Here's how the part is built. I have some questions about the finished solid (model axes, mm). Round coordinates to 2 decimals unless told otherwise and drop trailing zeros. Loops run counter-clockwise (first coordinate to the right, second up) from the corner with the lowest first, then second, coordinate; pieces in that order, holes last. Notation, with made-up numbers: M -5,-28 L 25,-28 A13 ccw 25,-3 Z; hole C 85.25,-36 d4. An arc over 180 degrees is marked long. Answer as a JSON object with one key per item and string values.
from build123d import *

# Parameters (mm, degrees)
F0_R     = 4.7625
F1_DEPTH = 58.166
F2_R     = 2.0828
F3_DEPTH = 11.43
F5_R     = 1.1811
F6_DEPTH = 10.16
F7_SIZE  = 0.762


with BuildPart() as f1:
    # F0 (on Front) → F1 (new body)
    with BuildSketch(Plane.XZ):
        Circle(F0_R)
    extrude(amount=F1_DEPTH)

    # F2 (on face) → F3 (cut)
    with BuildSketch(Plane.XZ.offset(58.166)):
        Circle(F2_R)
    extrude(amount=-F3_DEPTH, mode=Mode.SUBTRACT)

    # F5 (on offset) → F6 (cut)
    with BuildSketch(Plane.YZ.offset(4.7879)):
        with Locations((-3.175, 0)):
            Circle(F5_R)
    extrude(amount=-F6_DEPTH, mode=Mode.SUBTRACT)

    # F7
    f7_edges = [f1.edges().sort_by_distance(p)[0] for p in [
        (-4.7625, 0, 0),
    ]]
    chamfer(f7_edges, length=F7_SIZE)


solid = f1.part
Item 1: For P1, Ø2, axis at x = 3.5, y = -16.5, coming from the +Z side; P2, Ø3.5, axis at x = 0, z = 0, coming from the -Y side; P3, Ø1.5, axis at x = -1, y = -21.5, coming from the +Z side, each with a flat end and sliding along its axis, tell me the tip position at first contact or that it passes through.
Solution:
{"P1": "stops at z = 4.05", "P2": "stops at y = -46.74", "P3": "stops at z = 4.76"}
Item 2: I want a section at A-A on z = 0. List the corners of the cut face in (x, y) for me, plus the area to 3 significant figures.
Solution:
{"outline": "M -4.76,-58.17 L -2.08,-58.17 L -2.08,-46.74 L 2.08,-46.74 L 2.08,-58.17 L 4.76,-58.17 L 4.76,-4.36 L -4.76,-4.36 Z; M -4.76,-1.99 L 4.76,-1.99 L 4.76,-0.76 L 4,0 L -4,0 L -4.76,-0.76 Z", "area": "483 mm2"}
Item 3: If I drill on L1, parallel to Y at x = 0.5, z = 0; L2, parallel to Z at x = -0.25, y = -25.5; L3, parallel to Z at x = 0, y = -49, over which ranges is the centre line in solid material (lowest first)? Write a range as from..to.
Solution:
{"L1": "y = -46.74..-4.36, -1.99..0", "L2": "z = -4.76..4.76", "L3": "z = -4.76..-2.08, 2.08..4.76"}
Item 4: I want a section at B-B on x = 0. List the corners of the cut face in (y, z) for me (1 decimal).
Solution:
{"outline": "M -58.2,-4.8 L -0.8,-4.8 L 0,-4 L 0,4 L -0.8,4.8 L -58.2,4.8 L -58.2,2.1 L -46.7,2.1 L -46.7,-2.1 L -58.2,-2.1 Z; hole C -3.2,0 d2.4"}
Item 5: We'd pull the mould along Y, two halves only. Please class faces 1 (the face through (0.067, -2.048, 0.355)), 2 (the face through (1.987, -52.531, 0.626)), 3 (the face through (0, -46.736, 0)), 4 (the face through (0, 0, 0)): +Y half, -Y half, draft (parallel to the pull), parting line (faces both ways), or undercut.
Solution:
{"face 1": "undercut", "face 2": "draft", "face 3": "-Y half", "face 4": "+Y half"}
Item 6: I want a section at C-C on y = -48. List the corners of the cut face in (x, z) for me (1 decimal), plus the area to 3 significant figures.
Solution:
{"outline": "C 0,0 d9.5; hole C 0,0 d4.2", "area": "57.6 mm2"}
Item 7: I want a section at D-D on y = -25. List the corners of the cut face in (x, z) for me (1 decimal), plus the area to 3 significant figures.
Solution:
{"outline": "C 0,0 d9.5", "area": "71.3 mm2"}
